For this review, take the finished solid that the model builds, in its own axes (mm). A direction names the side the tool comes from. Round coordinates to 2 decimals unless told otherwise and drop trailing zeros. Write each loop counter-clockwise with the first axis right and the second up, starting at its lowest first coordinate (ties: lowest second). Pieces come first, ordered by that corner, then holes.
from build123d import *

# Parameters (mm, degrees)
SKETCH1_W           = 49
SKETCH1_H           = 21
SKETCH1_R           = 1
BOSS_EXTRUDE4_DEPTH = 10
CHAMFER2_SIZE       = 1
FILLET2_R           = 2
SKETCH2_W           = 49
SKETCH2_H           = 10
BOSS_EXTRUDE5_DEPTH = 30
CUT_EXTRUDE1_DEPTH  = 73
SKETCH4_3_R         = 80.5
SKETCH4_3_R_2       = 61.5
CUT_EXTRUDE2_DEPTH  = 5
SKETCH4_4_W         = 0.8
SKETCH4_4_H         = 8
CUT_EXTRUDE3_DEPTH  = 1
FILLET4_R           = 1.5
FILLET6_R           = 1.5
FILLET7_R           = 1


with BuildPart() as part:
    # Sketch1 → Boss-Extrude4 (new body)
    with BuildSketch(Plane.XY):
        with Locations((3.999954481, 0.020373254)):
            Rectangle(SKETCH1_W, SKETCH1_H)
        with Locations((-16.000045519, 0.020373254)):
            Circle(SKETCH1_R, mode=Mode.SUBTRACT)
        with Locations((-6.000045519, 0.020373254)):
            Circle(SKETCH1_R, mode=Mode.SUBTRACT)
        with Locations((13.999954481, -4.979626746)):
            Circle(SKETCH1_R, mode=Mode.SUBTRACT)
        with Locations((23.999954481, -4.979626746)):
            Circle(SKETCH1_R, mode=Mode.SUBTRACT)
        with Locations((-16.000045519, 5.020373254)):
            Circle(SKETCH1_R, mode=Mode.SUBTRACT)
        with Locations((3.999954481, 0.020373254)):
            Circle(SKETCH1_R, mode=Mode.SUBTRACT)
        with Locations((-6.000045519, 5.020373254)):
            Circle(SKETCH1_R, mode=Mode.SUBTRACT)
        with Locations((13.999954481, 0.020373254)):
            Circle(SKETCH1_R, mode=Mode.SUBTRACT)
        with Locations((23.999954481, 0.020373254)):
            Circle(SKETCH1_R, mode=Mode.SUBTRACT)
    extrude(amount=BOSS_EXTRUDE4_DEPTH)

    # Chamfer2
    chamfer2_edges = [part.edges().sort_by_distance(p)[0] for p in [
        (22.999954481, 0.020373254, 10),
        (12.999954481, 0.020373254, 10),
        (-17.000045519, 0.020373254, 10),
        (-7.000045519, 0.020373254, 10),
        (-17.000045519, 5.020373254, 10),
        (-7.000045519, 5.020373254, 10),
        (22.999954481, -4.979626746, 10),
        (12.999954481, -4.979626746, 10),
        (2.999954481, 0.020373254, 10),
    ]]
    chamfer(chamfer2_edges, length=CHAMFER2_SIZE)

    # Fillet2
    fillet2_edges = [part.edges().sort_by_distance(p)[0] for p in [
        (28.499954481, -10.479626746, 5),
        (-20.500045519, -10.479626746, 5),
    ]]
    fillet(fillet2_edges, radius=FILLET2_R)

    # Sketch2 → Boss-Extrude5 (add)
    with BuildSketch(Plane(origin=(0, 10.520373254, 0), x_dir=(1, 0, 0), z_dir=(0, 1, 0))):
        with Locations((3.999954481, -5)):
            Rectangle(SKETCH2_W, SKETCH2_H)
    extrude(amount=BOSS_EXTRUDE5_DEPTH)

    # Sketch4 → Cut-Extrude1 (cut)
    with BuildSketch(Plane.XY.offset(10)):
        with BuildLine():
            ThreePointArc((22.358468593, 22.87149124), (4.499954481, 20.520373254), (-13.358559631, 22.87149124))
            Line((-13.358559631, 22.87149124), (-14.393835812, 19.007787935))
            ThreePointArc((-14.393835812, 19.007787935), (4.499954481, 16.520373254), (23.393744773, 19.007787935))
            Line((23.393744773, 19.007787935), (22.358468593, 22.87149124))
        make_face()
        with BuildLine():
            Line((-20.500045519, 40.520373254), (-20.500045519, 37.739585311))
            ThreePointArc((-20.500045519, 37.739585311), (3.947268557, 32.023029505), (28.499954481, 37.268579027))
            Line((28.499954481, 37.268579027), (28.499954481, 40.520373254))
            Line((28.499954481, 40.520373254), (-20.500045519, 40.520373254))
        make_face()
        with BuildLine():
            ThreePointArc((61.999954481, 89.520373254), (-26.067593671, 138.222272601), (-20.500045519, 37.739585311))
            Line((-20.500045519, 37.739585311), (-20.500045519, 40.520373254))
            Line((-20.500045519, 40.520373254), (28.499954481, 40.520373254))
            Line((28.499954481, 40.520373254), (28.499954481, 37.268579027))
            ThreePointArc((28.499954481, 37.268579027), (52.905790906, 58.486117987), (61.999954481, 89.520373254))
        make_face()
    extrude(amount=-CUT_EXTRUDE1_DEPTH, mode=Mode.SUBTRACT)

    # Sketch4_3 → Cut-Extrude2 (cut)
    with BuildSketch(Plane.XY.offset(10)):
        with Locations((4.499954481, 89.520373254)):
            Circle(SKETCH4_3_R)
        with Locations((4.499954481, 89.520373254)):
            Circle(SKETCH4_3_R_2, mode=Mode.SUBTRACT)
    extrude(amount=-CUT_EXTRUDE2_DEPTH, mode=Mode.SUBTRACT)

    # Sketch4_4 → Cut-Extrude3 (cut)
    with BuildSketch(Plane.XY.offset(10)):
        with BuildLine():
            ThreePointArc((11.914383036, 9.362552368), (11.515991772, 9.326700058), (11.117427278, 9.292827774))
            Line((11.117427278, 9.292827774), (11.466136864, 5.307058968))
            Line((11.466136864, 5.307058968), (12.263092622, 5.376783563))
            Line((12.263092622, 5.376783563), (11.914383036, 9.362552368))
        make_face()
        with BuildLine():
            Line((-16.9838845, 7.796113315), (-15.948351106, 11.660776552))
            ThreePointArc((-15.948351106, 11.660776552), (-16.33497865, 11.763344238), (-16.721091767, 11.867831788))
            Line((-16.721091767, 11.867831788), (-17.756625161, 8.003168551))
            Line((-17.756625161, 8.003168551), (-16.9838845, 7.796113315))
        make_face()
        with BuildLine():
            ThreePointArc((-16.721091767, 11.867831788), (-16.33497865, 11.763344238), (-15.948351106, 11.660776552))
            Line((-15.948351106, 11.660776552), (-14.913332139, 15.523519925))
            Line((-14.913332139, 15.523519925), (-15.6860728, 15.730575161))
            Line((-15.6860728, 15.730575161), (-16.721091767, 11.867831788))
        make_face()
        Polygon((24.685981762, 15.730575161), (26.756534123, 8.003168551), (25.983793462, 7.796113315), (23.913241101, 15.523519925), align=None)
        Polygon((18.177963174, 14.25203942), (19.567148595, 6.373577396), (18.779302393, 6.234658854), (17.390116971, 14.113120878), align=None)
        with Locations((4.499954481, 9.020373254)):
            Rectangle(SKETCH4_4_W, SKETCH4_4_H)
        Polygon((-1.76898196, 13.276616553), (-2.466227902, 5.307058968), (-3.26318366, 5.376783563), (-2.565937719, 13.346341147), align=None)
        Polygon((-8.390208009, 14.113120878), (-9.779393431, 6.234658854), (-10.567239633, 6.373577396), (-9.178054212, 14.25203942), align=None)
    extrude(amount=-CUT_EXTRUDE3_DEPTH, mode=Mode.SUBTRACT)

    # Fillet4
    fillet4_edges = [part.edges().sort_by_distance(p)[0] for p in [
        (-13.358559631, 22.87149124, 2.5),
        (22.358468593, 22.87149124, 2.5),
        (23.393744773, 19.007787935, 2.5),
        (-14.393835812, 19.007787935, 2.5),
    ]]
    fillet(fillet4_edges, radius=FILLET4_R)

    # Fillet6
    fillet6_edges = [part.edges().sort_by_distance(p)[0] for p in [
        (28.499954481, 37.268579027, 5),
        (-20.500045519, 37.739585311, 5),
    ]]
    fillet(fillet6_edges, radius=FILLET6_R)

    # Fillet7
    fillet7_edges = [part.edges().sort_by_distance(p)[0] for p in [
        (-20.500045519, 13.000767923, 7.5),
        (-20.500045519, 33.33096144, 7.5),
        (28.499954481, 32.89661499, 7.5),
        (28.499954481, 12.681255612, 7.5),
    ]]
    fillet(fillet7_edges, radius=FILLET7_R)


solid = part.part
(1) We need section D-D, the plane y = 14.5. Give the boundary of the cut face in (x, z).
Geometry check:
outline: (-20.5, 0) - (28.5, 0) - (28.5, 5) - (-20.5, 5) - close
(2) For pin 1 Ø1.4 at (x, y) = (-17, 10.5) entering from +Z; pin 2 Ø5 at (x, y) = (22, 27) entering from +Z; pin 3 Ø1 at (x, z) = (20.5, 5.5) entering from +Y; pin 4 Ø1 at (x, z) = (-7.5, 7) entering from +Y, all flat-tipped, find the tip position at first contact; note any pin that passes through.
Geometry check:
pin 1: stops at z = 10
pin 2: stops at z = 5
pin 3: stops at y = 34.44
pin 4: stops at y = 33.4
(3) Mouldability with a two-part tool opening along X and no side actions: class faces 4 (the face through (3.605, 28.027, 7.535)), 5 (the face through (-17, 5, 4)), 6 (the face through (-20.5, 8, 4)), 7 (the face through (27.9, -9.91, 5.07)) as pulls with the +X half, pulls with the -X half, needs draft (parallel to the pull), parting line crosses it, or undercut.
Geometry check:
face 4: parting line crosses it
face 5: undercut
face 6: pulls with the -X half
face 7: pulls with the +X half
(4) For line 1 along X through (y, z) = (-5, 3.75); line 2 along X through (y, z) = (5.5, 4.75); line 3 along Y through (x, z) = (-2, 4), list the stretches that pass through material, from the lowest coordinate up.
Geometry check:
line 1: x = -20.5 to 13, 15 to 23, 25 to 28.5
line 2: x = -20.5 to -16.88, -15.12 to -6.88, -5.12 to 28.5
line 3: y = -10.48 to 16.81, 20.83 to 32.39
(5) We need section A-A, the plane z = 6.75. State how many separate pieces and enclosed holes the cut face has, and give its area (3 significant figures).
Geometry check:
separate pieces: 2
enclosed holes: 9
area: 1,190 mm2
(6) We need section B-B, the plane x = -1. Give the boundary of the cut face in (y, z), and give its area (3 significant figures).
Geometry check:
outline: (-10.48, 0) - (16.73, 0) - (16.73, 5) - (9.21, 5) - (9.21, 10) - (-10.48, 10) - close; (20.74, 0) - (32.28, 0) - (32.28, 10) - (28.27, 10) - (28.27, 5) - (20.74, 5) - close
area: 312 mm2
(7) For faces 1 (the face through (4.25, 16.52, 2.54)), 2 (the face through (3.648, 32.027, 5.07)), 3 (the face through (11.7, 7.4, 9)), list the 3-axis set-ups (+Z, -Z, +X, -X, +Y, -Y) from which the entire face can be reached by the end or side of a thin tool; tool diameter is ignored.
Geometry check:
face 1: +Z, -Z
face 2: +Z, -Z, +Y
face 3: +Z
